Could you check a few things on this model? Use its own coordinates, in mm. A direction names the side the tool comes from. Round coordinates to 2 decimals unless told otherwise and drop trailing zeros. Loops run counter-clockwise (first coordinate to the right, second up) from the corner with the lowest first, then second, coordinate; pieces in that order, holes last. Notation, with made-up numbers: (2, 23.25) -> (55, 23.25) arc R24 ccw to (55, 55.25) -> close; hole circle Ø5 at (53, 78.5). An arc over 180 degrees is marked (long way). Put each result on its own line as item: value. Start each with the question number.
1. Imagine slicing it at B-B, the plane z = 36.5. Please give me the cut outline in (x, y).
2. Which directions (+Z, -Z, +X, -X, +Y, -Y) give clear straight access to the entire face, cutting with the end or side of a thin tool? Please do faces 1 (the flat face through (107, 52, 88)), 2 (the cylindrical face through (128.464, 19.589, 44.465)), 3 (the flat face through (129, 9, 44)).
3. Imagine slicing it at D-D, the plane y = 31.5. Please give me the cut outline in (x, z), and give its area (3 significant figures).
4. Imagine slicing it at C-C, the plane x = 83. Please give me the cut outline in (y, z), and give its area (3 significant figures).
5. I need wall thicknesses on line 1 (Y direction, x = 92.8, z = 5.5); line 2 (Z direction, x = 108, y = 62); line 3 (Y direction, x = 108.25, z = 21). Which ranges of each line are inside material? Lowest first, please. Write a range as [from, to].
6. If we mould it in two halves opening along Z, with no side actions, what happens to faces 4 (the flat face through (94, 16, 31)), 5 (the cylindrical face through (107.07, 69.434, 77.294)), 6 (the cylindrical face through (92.028, 18.394, 30.92)), 7 (the cylindrical face through (107.07, 62.392, 76.495))? For each: pulls with the +Z half, pulls with the -Z half, needs draft (parallel to the pull), parting line crosses it, or undercut.
7. Imagine slicing it at A-A, the plane y = 10.5. Please give me the cut outline in (x, z).
8. I'm going to push flat-ended pins straight in: P1, Ø2.5, axis at x = 106.5, z = 44, coming from the -Y side; P2, Ø5.5, axis at x = 103.5, y = 2.5, coming from the +Z side; P3, Ø6, axis at y = 17, z = 34.5, coming from the +X side. Where does each tip first touch, or does it pass through?
```python
from build123d import *

# Parameters (mm, degrees)
SKETCH1_W            = 94
SKETCH1_H            = 42
BOSS_EXTRUDE1_DEPTH  = 3
SKETCH2_W            = 4
SKETCH2_H            = 42
BOSS_EXTRUDE2_DEPTH  = 47
SKETCH3_R            = 12.5
SKETCH3_R_2          = 1.6
CUT_EXTRUDE1_DEPTH   = 114.176852757
SKETCH4_W            = 42
SKETCH4_H            = 5
BOSS_EXTRUDE3_DEPTH  = 40
SKETCH5_W            = 42
SKETCH5_H            = 5
BOSS_EXTRUDE4_DEPTH  = 38
SKETCH7_W            = 42
SKETCH7_H            = 42
SKETCH7_W_2          = 44
BOSS_EXTRUDE6_DEPTH  = 5
SKETCH9_R            = 2.15
CUT_EXTRUDE2_DEPTH   = 149.731301346
SKETCH11_W           = 10
SKETCH11_H           = 18
BOSS_EXTRUDE7_DEPTH  = 20
SKETCH13_R           = 5.5
CUT_EXTRUDE3_DEPTH   = 169.988165266
BOSS_EXTRUDE11_DEPTH = 5
SKETCH23_W           = 10
SKETCH23_H           = 26
BOSS_EXTRUDE12_DEPTH = 50
CUT_EXTRUDE7_DEPTH   = 193.595430891
SKETCH25_W           = 10
SKETCH25_H           = 18
BOSS_EXTRUDE13_DEPTH = 20
SKETCH26_R           = 5.5
CUT_EXTRUDE8_DEPTH   = 193.595430891
SKETCH27_W           = 12
SKETCH27_H           = 18
BOSS_EXTRUDE14_DEPTH = 69
CUT_EXTRUDE10_START  = -5
SKETCH28_R           = 5.5
CUT_EXTRUDE10_DEPTH  = 5
SKETCH29_R           = 5.5
CUT_EXTRUDE11_DEPTH  = 5
FILLET4_R            = 9
FILLET3_R            = 3
SKETCH30_W           = 91
SKETCH30_H           = 42
CUT_EXTRUDE12_DEPTH  = 181.413414135
SKETCH31_W           = 40
SKETCH31_H           = 0.3
CUT_EXTRUDE13_DEPTH  = 42


# Some blends are built 0.0001 mm under size
with BuildPart() as part:
    # Sketch1 → Boss-Extrude1 (new body)
    with BuildSketch(Plane(origin=(0, 0, 0), x_dir=(1, 0, 0), z_dir=(0, 1, 0))):
        with Locations((47, -21)):
            Rectangle(SKETCH1_W, SKETCH1_H)
    extrude(amount=BOSS_EXTRUDE1_DEPTH)

    # Sketch2 → Boss-Extrude2 (add)
    with BuildSketch(Plane.XZ):
        with Locations((2, 21)):
            Rectangle(SKETCH2_W, SKETCH2_H)
        with Locations((92, 21)):
            Rectangle(SKETCH2_W, SKETCH2_H)
    extrude(amount=-BOSS_EXTRUDE2_DEPTH)

    # Sketch3 → Cut-Extrude1 (cut, through all)
    with BuildSketch(Plane(origin=(94, 0, 0), x_dir=(0, 0, -1), z_dir=(1, 0, 0))):
        with Locations((-21, 26)):
            Circle(SKETCH3_R)
        with Locations((-36.5, 41.5)):
            Circle(SKETCH3_R_2)
        with Locations((-5.5, 41.5)):
            Circle(SKETCH3_R_2)
        with Locations((-36.5, 10.5)):
            Circle(SKETCH3_R_2)
        with Locations((-5.5, 10.5)):
            Circle(SKETCH3_R_2)
    extrude(amount=-CUT_EXTRUDE1_DEPTH, mode=Mode.SUBTRACT)

    # Sketch4 → Boss-Extrude3 (add)
    with BuildSketch(Plane(origin=(94, 0, 0), x_dir=(0, 0, -1), z_dir=(1, 0, 0))):
        with Locations((-21, 2.5)):
            Rectangle(SKETCH4_W, SKETCH4_H)
    extrude(amount=BOSS_EXTRUDE3_DEPTH)

    # Sketch5 → Boss-Extrude4 (add)
    with BuildSketch(Plane.ZY):
        with Locations((21, 2.5)):
            Rectangle(SKETCH5_W, SKETCH5_H)
    extrude(amount=BOSS_EXTRUDE4_DEPTH)

    # Sketch7 → Boss-Extrude6 (add)
    with BuildSketch(Plane(origin=(0, 47, 0), x_dir=(1, 0, 0), z_dir=(0, 1, 0))):
        with Locations((-17, -21)):
            Rectangle(SKETCH7_W, SKETCH7_H)
        with Locations((112, -21)):
            Rectangle(SKETCH7_W_2, SKETCH7_H)
    extrude(amount=BOSS_EXTRUDE6_DEPTH)

    # Sketch9 → Cut-Extrude2 (cut, through all)
    with BuildSketch(Plane(origin=(0, 3, 0), x_dir=(1, 0, 0), z_dir=(0, 1, 0))):
        with Locations(Location((83, -21, 0), (0, 0, 270))):
            Circle(SKETCH9_R)
        with Locations(Location((65, -21, 0), (0, 0, 270))):
            Circle(SKETCH9_R)
        with Locations(Location((74, -12, 0), (0, 0, 270))):
            Circle(SKETCH9_R)
        with Locations(Location((74, -30, 0), (0, 0, 270))):
            Circle(SKETCH9_R)
        with Locations(Location((22, -12, 0), (0, 0, 270))):
            Circle(SKETCH9_R)
        with Locations(Location((22, -30, 0), (0, 0, 270))):
            Circle(SKETCH9_R)
    extrude(amount=-CUT_EXTRUDE2_DEPTH, mode=Mode.SUBTRACT)

    # Sketch11 → Boss-Extrude7 (add)
    with BuildSketch(Plane(origin=(0, 52, 0), x_dir=(1, 0, 0), z_dir=(0, 1, 0))):
        with Locations((-8, -21)):
            Rectangle(SKETCH11_W, SKETCH11_H)
        with Locations((107, -21)):
            Rectangle(SKETCH11_W, SKETCH11_H)
    extrude(amount=BOSS_EXTRUDE7_DEPTH)

    # Sketch13 → Cut-Extrude3 (cut, through all)
    with BuildSketch(Plane.ZY.offset(13)):
        with Locations((21, 62.15)):
            Circle(SKETCH13_R)
    extrude(amount=-CUT_EXTRUDE3_DEPTH, mode=Mode.SUBTRACT)

    # Sketch20 → Boss-Extrude11 (add)
    with BuildSketch(Plane.XY.offset(42)):
        Polygon((134, 0), (134, 52), (90, 52), (90, 0), (95, 0), (95, 20), (102, 26), (112, 26), (129, 20), (129, 0), align=None)
    extrude(amount=BOSS_EXTRUDE11_DEPTH)

    # Sketch23 → Boss-Extrude12 (add)
    with BuildSketch(Plane.XY.offset(47)):
        with Locations((107, 39)):
            Rectangle(SKETCH23_W, SKETCH23_H)
    extrude(amount=BOSS_EXTRUDE12_DEPTH)

    # Sketch24 → Cut-Extrude7 (cut, through all)
    with BuildSketch(Plane(origin=(112, 0, 0), x_dir=(0, 0, -1), z_dir=(1, 0, 0))):
        Polygon((-47, 26), (-97, 39), (-97, 26), align=None)
    extrude(amount=-CUT_EXTRUDE7_DEPTH, mode=Mode.SUBTRACT)

    # Sketch25 → Boss-Extrude13 (add)
    with BuildSketch(Plane(origin=(0, 52, 0), x_dir=(1, 0, 0), z_dir=(0, 1, 0))):
        with Locations((107, -71)):
            Rectangle(SKETCH25_W, SKETCH25_H)
    extrude(amount=BOSS_EXTRUDE13_DEPTH)

    # Sketch26 → Cut-Extrude8 (cut, through all)
    with BuildSketch(Plane(origin=(112, 0, 0), x_dir=(0, 0, -1), z_dir=(1, 0, 0))):
        with Locations((-71, 62.15)):
            Circle(SKETCH26_R)
    extrude(amount=-CUT_EXTRUDE8_DEPTH, mode=Mode.SUBTRACT)

    # Sketch27 → Boss-Extrude14 (add)
    with BuildSketch(Plane(origin=(0, 3, 0), x_dir=(1, 0, 0), z_dir=(0, 1, 0))):
        with Locations((47, -21)):
            Rectangle(SKETCH27_W, SKETCH27_H)
    extrude(amount=BOSS_EXTRUDE14_DEPTH)

    # Sketch28 → Cut-Extrude10 (cut)
    with BuildSketch(Plane(origin=(53, 0, 0), x_dir=(0, 0, -1), z_dir=(1, 0, 0)).offset(CUT_EXTRUDE10_START)):
        with Locations(Location((-21, 62.15, 0), (0, 0, 180))):
            Circle(SKETCH28_R)
    extrude(amount=CUT_EXTRUDE10_DEPTH, mode=Mode.SUBTRACT)

    # Sketch29 → Cut-Extrude11 (cut)
    with BuildSketch(Plane.ZY.offset(-41)):
        with Locations((21, 62.15)):
            Circle(SKETCH29_R)
    extrude(amount=-CUT_EXTRUDE11_DEPTH, mode=Mode.SUBTRACT)

    # Fillet4
    fillet4_edges = [part.edges().sort_by_distance(p)[0] for p in [
        (-8, 72, 12),
        (-8, 72, 30),
        (107, 72, 12),
        (107, 72, 30),
        (107, 72, 62),
        (107, 72, 80),
        (47, 72, 12),
        (47, 72, 30),
    ]]
    fillet(fillet4_edges, radius=FILLET4_R - 0.0001)  # a hair under: the kernel refuses the full size

    # Fillet3
    # the kernel refuses this fillet: 3 mm, written as the material it adds along each edge
    with BuildSketch(Plane(origin=(-3, 52, 30), x_dir=(0, 1, 0), z_dir=(-1, 0, 0)), Plane(origin=(112, 52, 80), x_dir=(0, 1, 0), z_dir=(-1, 0, 0))) as fillet3_piece_1:
        with BuildLine():
            CenterArc((FILLET3_R, -FILLET3_R), FILLET3_R, 90, 90)
            Line((0, -FILLET3_R), (0, 0))
            Line((0, 0), (FILLET3_R, 0))
        make_face()
    extrude(amount=10)
    with BuildSketch(Plane(origin=(-13, 52, 12), x_dir=(0, 0, -1), z_dir=(1, 0, 0)), Plane(origin=(112, 52, 30), x_dir=(0, 0, 1), z_dir=(-1, 0, 0)), Plane(origin=(102, 52, 12), x_dir=(0, 0, -1), z_dir=(1, 0, 0)), Plane(origin=(102, 52, 62), x_dir=(0, 0, -1), z_dir=(1, 0, 0))) as fillet3_piece_2:
        with BuildLine():
            CenterArc((FILLET3_R, FILLET3_R), FILLET3_R, 180, 90)
            Line((0, FILLET3_R), (0, 0))
            Line((0, 0), (FILLET3_R, 0))
        make_face()
    extrude(amount=10)
    with BuildSketch(Plane(origin=(95, 20, 42), x_dir=(0, -1, 0), z_dir=(0, 0, 1))) as fillet3_piece_3:
        with BuildLine():
            CenterArc((FILLET3_R * 0.45993492247, FILLET3_R), FILLET3_R, 220.601294645, 49.398705355)
            Line((-FILLET3_R * 0.299321679895, FILLET3_R * 0.349208626544), (0, 0))
            Line((0, 0), (FILLET3_R * 0.45993492247, 0))
        make_face()
    extrude(amount=5)
    with BuildSketch(Plane(origin=(102, 26, 42), x_dir=(-0.7592566023652966, -0.6507913734559685, 0), z_dir=(0, 0, 1))) as fillet3_piece_4:
        with BuildLine():
            CenterArc((FILLET3_R * 0.369924076215, FILLET3_R), FILLET3_R, 229.398705355, 40.601294645)
            Line((-FILLET3_R * 0.28086729724, FILLET3_R * 0.240743397635), (0, 0))
            Line((0, 0), (FILLET3_R * 0.369924076215, 0))
        make_face()
    extrude(amount=5)
    with BuildSketch(Plane(origin=(112, 26, 42), x_dir=(0.942990333582889, -0.3328201177351389, 0), z_dir=(0, 0, 1))) as fillet3_piece_5:
        with BuildLine():
            CenterArc((FILLET3_R * 0.171292729553, -FILLET3_R), FILLET3_R, 90, 19.440034828)
            Line((-FILLET3_R * 0.161527388182, -FILLET3_R * 0.0570096664171), (0, 0))
            Line((0, 0), (FILLET3_R * 0.171292729553, 0))
        make_face()
    extrude(amount=5)
    with BuildSketch(Plane(origin=(129, 20, 42), x_dir=(0, -1, 0), z_dir=(0, 0, 1))) as fillet3_piece_6:
        with BuildLine():
            CenterArc((FILLET3_R * 0.707515081019, -FILLET3_R), FILLET3_R, 90, 70.559965172)
            Line((-FILLET3_R * 0.235475252564, -FILLET3_R * 0.667179882265), (0, 0))
            Line((0, 0), (FILLET3_R * 0.707515081019, 0))
        make_face()
    extrude(amount=5)
    with BuildSketch(Plane(origin=(53, 3, 30), x_dir=(0, 0, 1), z_dir=(-1, 0, 0)), Plane(origin=(41, 3, 12), x_dir=(0, 0, -1), z_dir=(1, 0, 0))) as fillet3_piece_7:
        with BuildLine():
            CenterArc((FILLET3_R, FILLET3_R), FILLET3_R, 180, 90)
            Line((0, FILLET3_R), (0, 0))
            Line((0, 0), (FILLET3_R, 0))
        make_face()
    extrude(amount=12)
    # the kernel refuses this fillet: 3 mm, written as the material it takes off along each edge
    with BuildSketch(Plane(origin=(94.5, 52, 97), x_dir=(0, 0, -1), z_dir=(1, 0, 0))) as fillet3_2_piece_1:
        with BuildLine():
            CenterArc((FILLET3_R, -FILLET3_R), FILLET3_R, 90, 90)
            Line((0, -FILLET3_R), (0, 0))
            Line((0, 0), (FILLET3_R, 0))
        make_face()
    extrude(amount=25, mode=Mode.SUBTRACT)
    with BuildSketch(Plane(origin=(117.799354812, 39, 97), x_dir=(0, -0.25163385176495195, -0.9678225067882716), z_dir=(-1, 0, 0))) as fillet3_2_piece_2:
        with BuildLine():
            CenterArc((FILLET3_R * 0.773247308247, -FILLET3_R), FILLET3_R, 90, 75.425783802)
            Line((-FILLET3_R * 0.194575198541, -FILLET3_R * 0.748366148235), (0, 0))
            Line((0, 0), (FILLET3_R * 0.773247308247, 0))
        make_face()
    extrude(amount=21.598709624, mode=Mode.SUBTRACT)

    # Sketch30 → Cut-Extrude12 (cut, through all)
    with BuildSketch(Plane.XZ):
        with Locations((7.5, 21)):
            Rectangle(SKETCH30_W, SKETCH30_H)
    extrude(amount=-CUT_EXTRUDE12_DEPTH, mode=Mode.SUBTRACT)

    # Sketch31 → Cut-Extrude13 (cut)
    with BuildSketch(Plane(origin=(0, 0, 0), x_dir=(-1, 0, 0), z_dir=(0, 0, -1))):
        with Locations((-114, 47.15)):
            Rectangle(SKETCH31_W, SKETCH31_H)
    extrude(amount=-CUT_EXTRUDE13_DEPTH, mode=Mode.SUBTRACT)


solid = part.part
```
Entries:
1. outline: (53, 0) -> (134, 0) -> (134, 5) -> (94, 5) -> (94, 8.9) -> (90, 8.9) -> (90, 3) -> (53, 3) -> close; (90, 12.1) -> (94, 12.1) -> (94, 39.9) -> (90, 39.9) -> close; (90, 43.1) -> (94, 43.1) -> (94, 47.3) -> (134, 47.3) -> (134, 52) -> (90, 52) -> close
2. face 1: +Z, +X, -X, +Y
2. face 2: +Z, -Z, -Y
2. face 3: +Z, -Y
3. outline: (90, 0) -> (94, 0) -> (94, 9.78) -> (90, 9.78) -> close; (90, 32.22) -> (94, 32.22) -> (94, 42) -> (134, 42) -> (134, 47) -> (112, 47) -> (112, 68.15) -> (102, 68.15) -> (102, 47) -> (90, 47) -> close
3. area: 510 mm^2
4. outline: (0, 0) -> (3, 0) -> (3, 18.85) -> (0, 18.85) -> close; (0, 23.15) -> (3, 23.15) -> (3, 42) -> (0, 42) -> close
4. area: 113 mm^2
5. line 1: [0, 8.9], [12.1, 39.9], [43.1, 52]
5. line 2: [12, 15.5], [26.5, 30], [62, 65.5], [76.5, 80]
5. line 3: [0, 5], [47.3, 56.65], [67.65, 72]
6. face 4: needs draft
6. face 5: pulls with the +Z half
6. face 6: undercut
6. face 7: undercut
7. outline: (90, 0) -> (94, 0) -> (94, 3.9) -> (90, 3.9) -> close; (90, 7.1) -> (94, 7.1) -> (94, 34.9) -> (90, 34.9) -> close; (90, 38.1) -> (94, 38.1) -> (94, 42) -> (95, 42) -> (95, 47) -> (90, 47) -> close; (129, 42) -> (134, 42) -> (134, 47) -> (129, 47) -> close
8. P1: y = 26
8. P2: z = 42
8. P3: x = 94
